The model under review builds one solid part; all positions refer to its coordinate system, in mm. Round coordinates to 2 decimals unless told otherwise and drop trailing zeros. Write each loop counter-clockwise with the first axis right and the second up, starting at its lowest first coordinate (ties: lowest second). Pieces come first, ordered by that corner, then holes. Notation, with made-up numbers: (22.5, 66.25) - (57.5, 66.25) arc R18 cw to (57.5, 99.25) - close; hole circle Ø7 at (20.25, -6.75). An arc over 180 degrees is marked (long way). Return JSON: item names as keys, results as strings.
from build123d import *

# Parameters (mm, degrees)
SKETCH1_R           = 15
EXTRUDE1_DEPTH      = 8
SKETCH2_R           = 12
EXTRUDE2_DEPTH      = 170
EXTRUDE3_DEPTH      = 172.31841699
EXTRUDE3_DEPTH_BACK = 172.31841699
SKETCH3_R           = 4
CHAMFER1_SIZE       = 2


with BuildPart() as part:
    # Sketch1 → Extrude1 (new body)
    with BuildSketch(Plane(origin=(0, 0, 0), x_dir=(1, 0, 0), z_dir=(0, 1, 0))):
        with Locations(Location((0, 0, 0), (0, 0, 270))):
            Circle(SKETCH1_R)
    extrude(amount=EXTRUDE1_DEPTH)

    # Sketch2 → Extrude2 (add)
    with BuildSketch(Plane.XZ):
        with Locations(Location((0, 0, 0), (0, 0, 270))):
            Circle(SKETCH2_R)
    extrude(amount=EXTRUDE2_DEPTH)

    # Sketch3 → Extrude3 (cut, two sides: drawn at the far end of the back side and taken through both)
    with BuildSketch(Plane(origin=(0, 0, 0), x_dir=(0, 0, -1), z_dir=(1, 0, 0)).offset(-EXTRUDE3_DEPTH_BACK)):
        with Locations((0, -162)):
            Circle(SKETCH3_R)
    extrude(amount=EXTRUDE3_DEPTH + EXTRUDE3_DEPTH_BACK, mode=Mode.SUBTRACT)

    # Chamfer1
    chamfer1_edges = [part.edges().sort_by_distance(p)[0] for p in [
        (0, 8, -15),
        (0, -170, 12),
    ]]
    chamfer(chamfer1_edges, length=CHAMFER1_SIZE)


solid = part.part
(1) Clearance check with flat-ended pins moving along their axes: pin 1 Ø1.5 at (x, y) = (-10.5, -129.5) entering from +Z; pin 2 Ø1.5 at (x, y) = (-11, -37) entering from -Z; pin 3 Ø12 at (x, y) = (-8.5, -41) entering from +Z; pin 4 Ø6.5 at (y, z) = (-162, 0) entering from -X. State where each tip first meets the part, or that it passes through.
Filled in:
{"pin 1": "stops at z = 7", "pin 2": "stops at z = -6.24", "pin 3": "stops at z = 11.74", "pin 4": "passes through"}
(2) Mouldability with a two-part tool opening along Y and no side actions: class faces 1 (the flat face through (0, -170, 0)), 2 (the cylindrical face through (-0.168, -158.034, 0.521)), 3 (the cylindrical face through (0.66, 2.958, -14.985)), 4 (the flat face through (0, 8, 0)) as released by +Y, released by -Y, zero draft, split by the parting line, or undercut.
Filled in:
{"face 1": "released by -Y", "face 2": "undercut", "face 3": "zero draft", "face 4": "released by +Y"}
(3) Add section B-B (z = 0). Write out the cut boundary in (x, y).
Filled in:
{"outline": "(-15, 0) - (-12, 0) - (-12, -158) - (12, -158) - (12, 0) - (15, 0) - (15, 6) - (13, 8) - (-13, 8) - (-15, 6) - close; (-12, -168) - (-10, -170) - (10, -170) - (12, -168) - (12, -166) - (-12, -166) - close"}
(4) Add section A-A (x = 0). Write out the cut boundary in (y, z).
Filled in:
{"outline": "(-170, -10) - (-168, -12) - (0, -12) - (0, -15) - (6, -15) - (8, -13) - (8, 13) - (6, 15) - (0, 15) - (0, 12) - (-168, 12) - (-170, 10) - close; hole circle Ø8 at (-162, 0)"}
(5) Wall thickness on line 1 (Y direction, x = -6.5, z = 0); line 2 (X direction, y = -83, z = -0.25); line 3 (Z direction, x = 5, y = -162): over which ranges is each line inside the solid? List them lowest first.
Filled in:
{"line 1": "y = -170 to -166, -158 to 8", "line 2": "x = -12 to 12", "line 3": "z = -10.91 to -4, 4 to 10.91"}
(6) Add section D-D (y = -162). Write out the cut boundary in (x, z).
Filled in:
{"outline": "(-11.31, -4) arc R12 ccw to (11.31, -4) - close; (-11.31, 4) - (11.31, 4) arc R12 ccw to start"}
(7) Add section C-C (y = -61). Write out the cut boundary in (x, z).
Filled in:
{"outline": "circle Ø24 at (0, 0)"}
